Check sheet for the modelled part. Datum: model origin and axes. Units: mm. Face numbers are marked on the shaded views. A direction names the side the tool comes from. Give positions to 0.01 mm unless a question says otherwise; leave off trailing zeros. Order: outer loops, then holes, each group sorted by start corner. A loop starts at its lowest first (then second) coordinate and runs counter-clockwise, first axis right, second up.
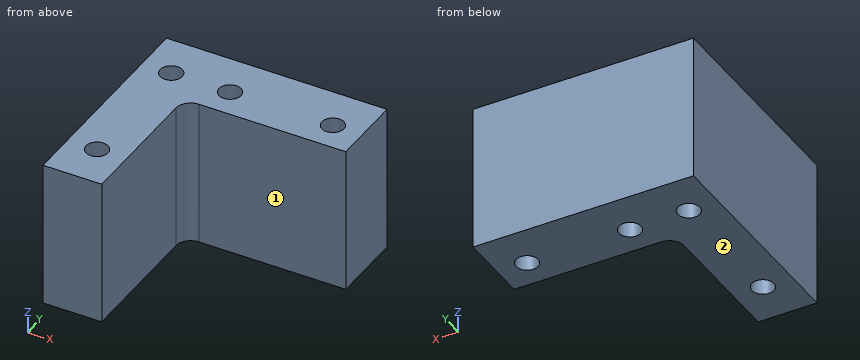
from build123d import *

# Parameters (mm, degrees)
SKETCH1_R           = 1.905
BOSS_EXTRUDE1_DEPTH = 25.4


with BuildPart() as part:
    # Sketch1 → Boss-Extrude1 (new body)
    with BuildSketch(Plane.XY):
        with BuildLine():
            Line((0, 0), (0, 38.1))
            Line((0, 38.1), (38.1, 38.1))
            Line((38.1, 38.1), (38.1, 25.4))
            Line((38.1, 25.4), (12.7, 25.4))
            ThreePointArc((12.7, 25.4), (10.903948776, 24.656051224), (10.16, 22.86))
            Line((10.16, 22.86), (10.16, 0))
            Line((10.16, 0), (0, 0))
        make_face()
        with Locations((5.08, 30.48)):
            Circle(SKETCH1_R, mode=Mode.SUBTRACT)
        with Locations((5.08, 7.62)):
            Circle(SKETCH1_R, mode=Mode.SUBTRACT)
        with Locations((15.24, 30.48)):
            Circle(SKETCH1_R, mode=Mode.SUBTRACT)
        with Locations((33.02, 30.48)):
            Circle(SKETCH1_R, mode=Mode.SUBTRACT)
    extrude(amount=BOSS_EXTRUDE1_DEPTH)


solid = part.part
1) Depth check by flat-ended pin: pin 1 Ø6 at (y, z) = (21.5, 4.5) entering from -X; pin 2 Ø1 at (x, y) = (32.5, 29.5) entering from +Z; pin 3 Ø8 at (x, z) = (17, 9.5) entering from -Y; pin 4 Ø2 at (y, z) = (17.5, 10.5) entering from +X. Enter the tip coordinate at first touch or a pass-through.
Recorded:
pin 1: stops at x = 0
pin 2: passes through
pin 3: stops at y = 25.4
pin 4: stops at x = 10.16
2) Section check C-C, the plane x = 5.08. Record the cut outline in (y, z) (3 decimals).
Recorded:
outline: (0, 0) - (5.715, 0) - (5.715, 25.4) - (0, 25.4) - close; (9.525, 0) - (28.575, 0) - (28.575, 25.4) - (9.525, 25.4) - close; (32.385, 0) - (38.1, 0) - (38.1, 25.4) - (32.385, 25.4) - close
3) Section check A-A, the plane x = 33.02. Record the cut outline in (y, z) (3 decimals).
Recorded:
outline: (25.4, 0) - (28.575, 0) - (28.575, 25.4) - (25.4, 25.4) - close; (32.385, 0) - (38.1, 0) - (38.1, 25.4) - (32.385, 25.4) - close
4) Section check D-D, the plane z = 15.5. Record the cut outline in (x, y) (3 decimals).
Recorded:
outline: (0, 0) - (10.16, 0) - (10.16, 22.86) arc R2.54 cw to (12.7, 25.4) - (38.1, 25.4) - (38.1, 38.1) - (0, 38.1) - close; hole circle Ø3.81 at (5.08, 7.62); hole circle Ø3.81 at (5.08, 30.48); hole circle Ø3.81 at (15.24, 30.48); hole circle Ø3.81 at (33.02, 30.48)
5) Set-up check for the marked faces 1 and 2: record each of +Z, -Z, +X, -X, +Y, -Y from which the full face is reachable in a straight line by a thin tool's end or side.
Recorded:
face 1: +Z, -Z, +X, -Y
face 2: -Z, +X, -X, +Y, -Y
6) Material ranges on L1, parallel to Y at x = 5.08, z = 19 (3 decimals); L2, parallel to Y at x = 15.24, z = 9.25 (3 decimals); L3, parallel to X at y = 12.5, z = 16.5, recorded low to high.
Recorded:
L1: y = 0 to 5.715, 9.525 to 28.575, 32.385 to 38.1
L2: y = 25.4 to 28.575, 32.385 to 38.1
L3: x = 0 to 10.16
7) Section check B-B, the plane y = 30.48. Record the cut outline in (x, z) (3 decimals), then the cut area to 3 significant figures.
Recorded:
outline: (0, 0) - (3.175, 0) - (3.175, 25.4) - (0, 25.4) - close; (6.985, 0) - (13.335, 0) - (13.335, 25.4) - (6.985, 25.4) - close; (17.145, 0) - (31.115, 0) - (31.115, 25.4) - (17.145, 25.4) - close; (34.925, 0) - (38.1, 0) - (38.1, 25.4) - (34.925, 25.4) - close
area: 677 mm2
